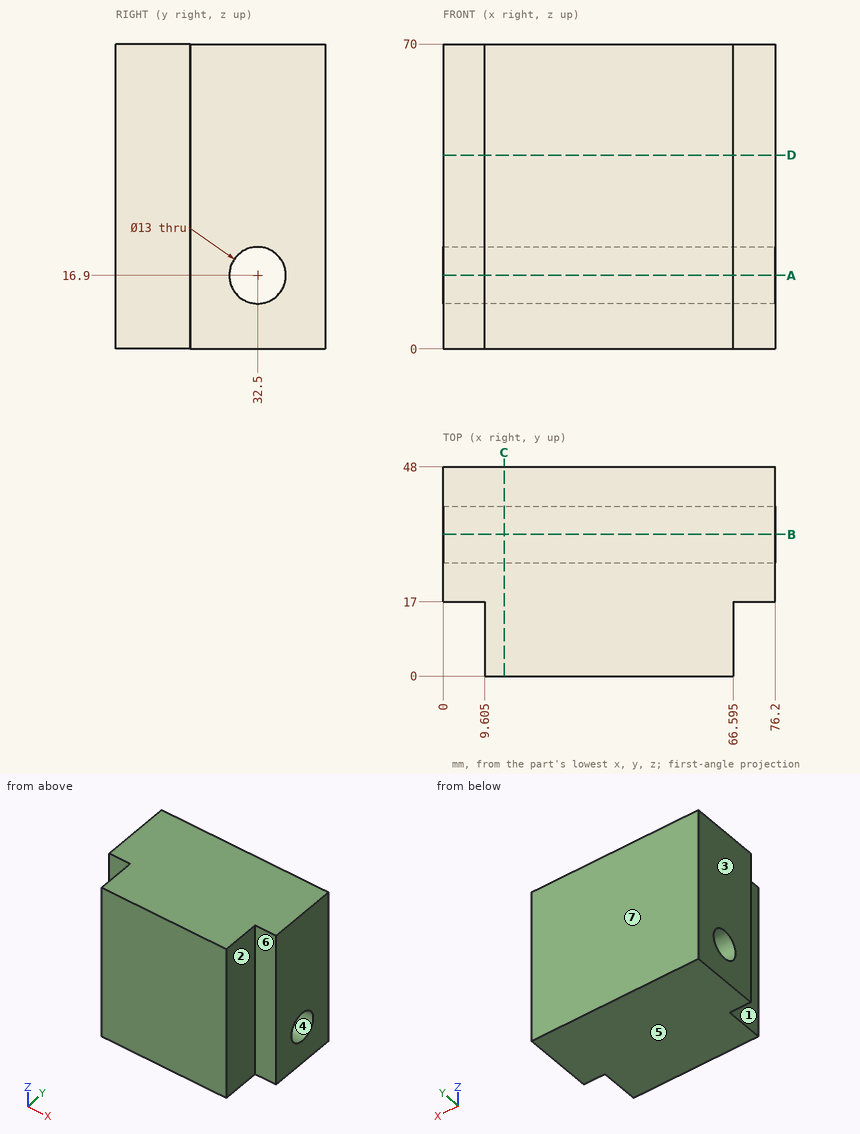
Here's the drawing with two shaded views (mm, measured from the low corner). I have some questions. A direction names the side the tool comes from. Give positions to 0.01 mm unless a question says otherwise; leave off trailing zeros. Loops run counter-clockwise (first coordinate to the right, second up) from the corner with the lowest first, then second, coordinate; pieces in that order, holes last. Notation, with made-up numbers: M 6,72 L 16,72 A16 ccw 16,90 Z; hole C -37,5 d1. An arc over 180 degrees is marked long. Use one line per item in the form item = value. Start each with the question number.
(1) I'm going to push flat-ended pins straight in: P1, Ø13.5, axis at y = 9.5, z = 28.5, coming from the +X side (1 decimal); P2, Ø3, axis at x = 5, z = 49, coming from the -Y side; P3, Ø1.5, axis at y = 6.5, z = 57, coming from the -X side (1 decimal). Where does each tip first touch, or does it pass through?
(2) Please list where these lines run through material, in increasing order: line 1 (Y direction, x = 59, z = 16.9); line 2 (Z direction, x = 58, y = 32); line 3 (X direction, y = 9, z = 15.5) (1 decimal).
(3) I want a section at C-C, the plane x = 14. Write out the boundary of the cut face in (y, z), and give its area (3 significant figures).
(4) On a 3-axis mill with a long thin cutter (end or side, diameter ignored), from which of +Z, -Z, +X, -X, +Y, -Y can I reach the whole of each face in a straight line? I mean the marked faces 1, 2 and 3. Say none if no direction works.
(5) I want a section at D-D, the plane z = 44.5. Write out the boundary of the cut face in (x, y) (1 decimal).
(6) Thinking about a two-plate mould opening in Y: for the marked faces 4, 5, 6 and 7, which applies, released by +Y, released by -Y, zero draft, split by the parting line, or undercut?
(7) I want a section at B-B, the plane y = 32.5. Write out the boundary of the cut face in (x, z), and give its area (3 significant figures).
(8) I want a section at A-A, the plane z = 16.9. Write out the boundary of the cut face in (x, y) (1 decimal), and give its area (3 significant figures).
Worked out:
q1.P1 = 66.6
q1.P2 = 17
q1.P3 = 9.6
q2.line_1 = 0 to 26, 39 to 48
q2.line_2 = 0 to 10.42, 23.38 to 70
q2.line_3 = 9.6 to 66.6
q3.outline = M 0,0 L 48,0 L 48,70 L 0,70 Z; hole C 32.5,16.9 d13
q3.area = 3,230 mm²
q4.face_1 = +Z, -Z, -X, -Y
q4.face_2 = +Z, -Z, +X, -Y
q4.face_3 = +Z, -Z, -X, +Y, -Y
q5.outline = M 0,17 L 9.6,17 L 9.6,0 L 66.6,0 L 66.6,17 L 76.2,17 L 76.2,48 L 0,48 Z
q6.face_4 = undercut
q6.face_5 = zero draft
q6.face_6 = released by -Y
q6.face_7 = released by +Y
q7.outline = M 0,0 L 76.2,0 L 76.2,10.4 L 0,10.4 Z; M 0,23.4 L 76.2,23.4 L 76.2,70 L 0,70 Z
q7.area = 4,340 mm²
q8.outline = M 0,17 L 9.6,17 L 9.6,0 L 66.6,0 L 66.6,17 L 76.2,17 L 76.2,26 L 0,26 Z; M 0,39 L 76.2,39 L 76.2,48 L 0,48 Z
q8.area = 2,340 mm²
